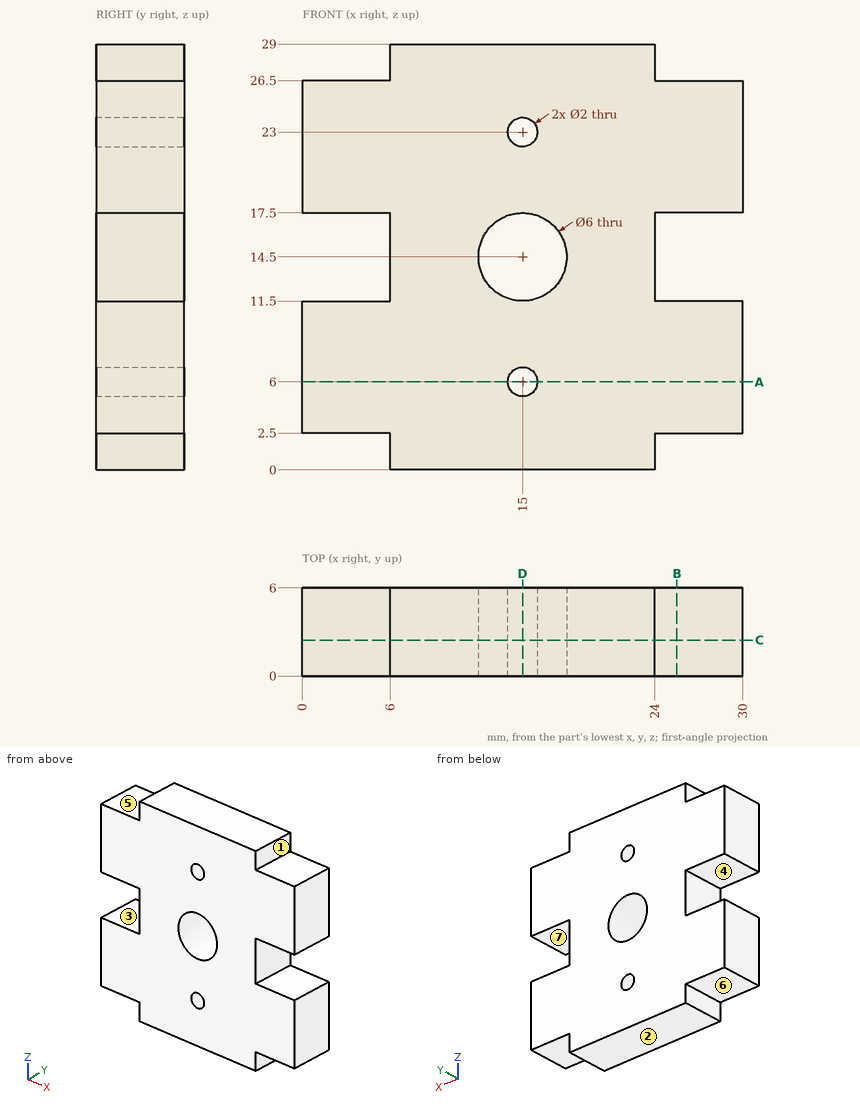
Answer from the drawing. Dimensions are ordinates in mm from the lowest x, y and z of the part. A direction names the side the tool comes from. Give positions to 0.01 mm unless a question says otherwise; leave off trailing zeros. Loops run counter-clockwise (first coordinate to the right, second up) from the corner with the lowest first, then second, coordinate; pieces in that order, holes last. Notation, with made-up numbers: (22.25, 13) - (65.25, 13) arc R21 cw to (65.25, 30) - close; hole circle Ø9 at (73, 79.5). An arc over 180 degrees is marked (long way). Answer as a JSON object with one key per item and string values.
1. Find the intervals of material crossed by L1, parallel to Z at x = 15, y = 4.5; L2, parallel to Z at x = 26.25, y = 4.75; L3, parallel to Z at x = 15.75, y = 1.8, in increasing order. Write a range as [from, to].
Determined:
{"L1": "[0, 5], [7, 11.5], [17.5, 22], [24, 29]", "L2": "[2.5, 11.5], [17.5, 26.5]", "L3": "[0, 5.34], [6.66, 11.6], [17.4, 22.34], [23.66, 29]"}
2. For the marked faces 4, 5, 6 and 7, determine the directions among +Z, -Z, +X, -X, +Y, -Y from which every point of the face is accessible in a straight line to the end or side of a thin tool.
Determined:
{"face 4": "-X, +Y, -Y", "face 5": "+Z, -X, +Y, -Y", "face 6": "-Z, -X, +Y, -Y", "face 7": "+X, +Y, -Y"}
3. For a pull along Z with two mould halves and no side action, classify the marked faces 1, 2 and 3 as pulls with the +Z half, pulls with the -Z half, needs draft (parallel to the pull), parting line crosses it, or undercut.
Determined:
{"face 1": "needs draft", "face 2": "pulls with the -Z half", "face 3": "undercut"}
4. A cutting plane is placed at A-A (z = 6). Write down the section's boundary in (x, y).
Determined:
{"outline": "(0, 0) - (14, 0) - (14, 6) - (0, 6) - close; (16, 0) - (30, 0) - (30, 6) - (16, 6) - close"}
5. A cutting plane is placed at B-B (x = 25.5). Write down the section's boundary in (y, z).
Determined:
{"outline": "(0, 2.5) - (6, 2.5) - (6, 11.5) - (0, 11.5) - close; (0, 17.5) - (6, 17.5) - (6, 26.5) - (0, 26.5) - close"}
6. A cutting plane is placed at D-D (x = 15). Write down the section's boundary in (y, z).
Determined:
{"outline": "(0, 0) - (6, 0) - (6, 5) - (0, 5) - close; (0, 7) - (6, 7) - (6, 11.5) - (0, 11.5) - close; (0, 17.5) - (6, 17.5) - (6, 22) - (0, 22) - close; (0, 24) - (6, 24) - (6, 29) - (0, 29) - close"}
7. A cutting plane is placed at C-C (y = 2.45). Write down the section's boundary in (x, z), then the cut area to 3 significant figures.
Determined:
{"outline": "(0, 2.5) - (6, 2.5) - (6, 0) - (24, 0) - (24, 2.5) - (30, 2.5) - (30, 11.5) - (24, 11.5) - (24, 17.5) - (30, 17.5) - (30, 26.5) - (24, 26.5) - (24, 29) - (6, 29) - (6, 26.5) - (0, 26.5) - (0, 17.5) - (6, 17.5) - (6, 11.5) - (0, 11.5) - close; hole circle Ø6 at (15, 14.5); hole circle Ø2 at (15, 6); hole circle Ø2 at (15, 23)", "area": "703 mm²"}
8. Flat-ended cylindrical pins translate along their axes: pin 1 Ø1.8 at (y, z) = (2, 14) entering from -X; pin 2 Ø1.8 at (x, y) = (27, 4.5) entering from +Z; pin 3 Ø3 at (y, z) = (1.5, 0.5) entering from +X. Find the tip coordinate at first contact, or state that the pin passes through.
Determined:
{"pin 1": "x = 6", "pin 2": "z = 26.5", "pin 3": "x = 24"}
